from build123d import *

# Parameters (mm, degrees)
SKIZZE1_W                       = 63
SKIZZE1_H                       = 54
AUFSATZ_LINEAR_AUSTRAGEN1_DEPTH = 4
SCHNITT_LINEAR_AUSTRAGEN3_REACH = 6
SKIZZE4_W                       = 9.5
SKIZZE4_H                       = 4
SKIZZE2_W                       = 5
SKIZZE2_H                       = 17.25
SKIZZE2_H_2                     = 21.25
SCHNITT_LINEAR_AUSTRAGEN1_DEPTH = 4
SKIZZE5_R                       = 8
SCHNITT_LINEAR_AUSTRAGEN4_DEPTH = 4


with BuildPart() as part:
    # Skizze1 → Aufsatz-Linear austragen1 (new body)
    with BuildSketch(Plane.XY):
        with Locations((31.5, 27)):
            Rectangle(SKIZZE1_W, SKIZZE1_H)
    extrude(amount=AUFSATZ_LINEAR_AUSTRAGEN1_DEPTH)

    # Skizze4 → Schnitt-Linear austragen3 (cut, up to next)
    with BuildSketch(Plane.XY.offset(4), mode=Mode.PRIVATE) as schnitt_linear_austragen3_sk1:
        with Locations((19.669225385, 2)):
            Rectangle(SKIZZE4_W, SKIZZE4_H)
    schnitt_linear_austragen3_tool1 = extrude(schnitt_linear_austragen3_sk1.sketch, amount=-SCHNITT_LINEAR_AUSTRAGEN3_REACH, mode=Mode.PRIVATE) & part.part
    add(schnitt_linear_austragen3_tool1.solids().sort_by_distance((19.669225, 2, 4))[0], mode=Mode.SUBTRACT)
    # Skizze4 → Schnitt-Linear austragen3 (cut, up to next)
    with BuildSketch(Plane.XY.offset(4), mode=Mode.PRIVATE) as schnitt_linear_austragen3_sk2:
        with Locations((42.669225385, 2)):
            Rectangle(SKIZZE4_W, SKIZZE4_H)
    schnitt_linear_austragen3_tool2 = extrude(schnitt_linear_austragen3_sk2.sketch, amount=-SCHNITT_LINEAR_AUSTRAGEN3_REACH, mode=Mode.PRIVATE) & part.part
    add(schnitt_linear_austragen3_tool2.solids().sort_by_distance((42.669225, 2, 4))[0], mode=Mode.SUBTRACT)

    # Skizze2 → Schnitt-Linear austragen1 (cut)
    with BuildSketch(Plane.XY.offset(4)):
        with Locations((2.5, 45.375)):
            Rectangle(SKIZZE2_W, SKIZZE2_H)
        with Locations((2.5, 10.625)):
            Rectangle(SKIZZE2_W, SKIZZE2_H_2)
    schnitt_linear_austragen1 = extrude(amount=-SCHNITT_LINEAR_AUSTRAGEN1_DEPTH, mode=Mode.SUBTRACT)

    # Spiegeln1: Schnitt-Linear austragen1 across plane
    add(schnitt_linear_austragen1.mirror(Plane.ZY.offset(-31.5)), mode=Mode.SUBTRACT)

    # Skizze5 → Schnitt-Linear austragen4 (cut)
    with BuildSketch(Plane.XY.offset(4)):
        with Locations((18, 34)):
            Circle(SKIZZE5_R)
        with BuildLine():
            Line((31.5, 43.55), (28.2, 43.55))
            ThreePointArc((28.2, 43.55), (26.2, 41.55), (28.2, 39.55))
            Line((28.2, 39.55), (31.5, 39.55))
            Line((31.5, 39.55), (31.5, 43.55))
        make_face()
    schnitt_linear_austragen4 = extrude(amount=-SCHNITT_LINEAR_AUSTRAGEN4_DEPTH, mode=Mode.SUBTRACT)

    # Spiegeln2: Schnitt-Linear austragen4 across plane
    add(schnitt_linear_austragen4.mirror(Plane.ZY.offset(-31.5)), mode=Mode.SUBTRACT)


solid = part.part
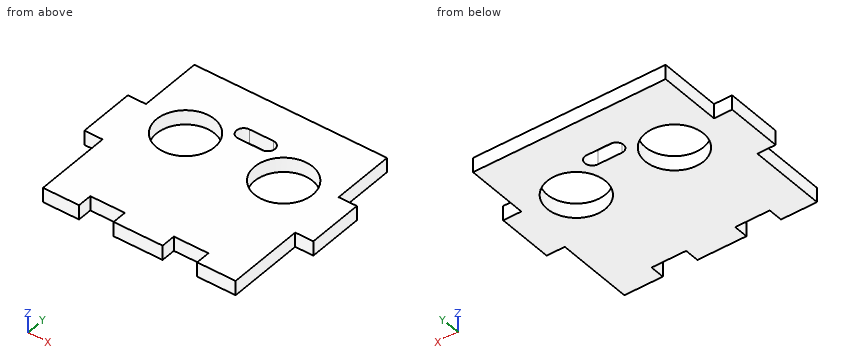
Part model, mm, in its own coordinate system. Give positions to 0.01 mm unless a question says otherwise; leave off trailing zeros. Loops run counter-clockwise (first coordinate to the right, second up) from the corner with the lowest first, then second, coordinate; pieces in that order, holes last. Notation, with made-up numbers: (-33, 77) -> (13, 77) arc R32 cw to (13, 111) -> close; hole circle Ø4 at (19, 0). An arc over 180 degrees is marked (long way). Write each question's results on one line, items separated by ' | '. Start each with the question number.
Q1. Band-saw the part on A-A on y = 34. List the corners of the cut face in (x, z).
Q2. Band-saw the part on D-D on x = 43.5. List the corners of the cut face in (y, z), plus the area to 3 significant figures.
Q3. Pin check, flat tips, straight feed: P1, Ø1.2, axis at y = 10, z = 2.5, coming from the -X side; P2, Ø2, axis at x = 17.5, z = 3, coming from the -Y side; P3, Ø1, axis at x = 51.5, y = 33, coming from the +Z side; P4, Ø2, axis at x = 3.5, z = 2.5, coming from the +Y side. Stop position of each tip, or through.
Q4. Wall check: L1, parallel to Y at x = 18, z = 2.3; L2, parallel to X at y = 31.5, z = 2.6; L3, parallel to X at y = 51.5, z = 0.2. Give the ranges that are in metal, low to high.
Q5. Band-saw the part on B-B on x = 18. List the corners of the cut face in (y, z), plus the area to 3 significant figures.
Q6. Band-saw the part on C-C on z = 1.75. List the corners of the cut face in (x, y).
Results are:
1) outline: (0, 0) -> (10, 0) -> (10, 4) -> (0, 4) -> close; (26, 0) -> (37, 0) -> (37, 4) -> (26, 4) -> close; (53, 0) -> (63, 0) -> (63, 4) -> (53, 4) -> close
2) outline: (4, 0) -> (26.14, 0) -> (26.14, 4) -> (4, 4) -> close; (41.86, 0) -> (54, 0) -> (54, 4) -> (41.86, 4) -> close | area: 137 mm²
3) P1: stops at x = 5 | P2: stops at y = 4 | P3: passes through | P4: stops at y = 36.75
4) L1: y = 4 to 26, 42 to 54 | L2: x = 0 to 10.4, 25.6 to 37.4, 52.6 to 63 | L3: x = 5 to 58
5) outline: (4, 0) -> (26, 0) -> (26, 4) -> (4, 4) -> close; (42, 0) -> (54, 0) -> (54, 4) -> (42, 4) -> close | area: 136 mm²
6) outline: (0, 21.25) -> (5, 21.25) -> (5, 0) -> (14.92, 0) -> (14.92, 4) -> (24.42, 4) -> (24.42, 0) -> (37.92, 0) -> (37.92, 4) -> (47.42, 4) -> (47.42, 0) -> (58, 0) -> (58, 21.25) -> (63, 21.25) -> (63, 36.75) -> (58, 36.75) -> (58, 54) -> (5, 54) -> (5, 36.75) -> (0, 36.75) -> close; hole circle Ø16 at (18, 34); hole (28.2, 39.55) -> (34.8, 39.55) arc R2 ccw to (34.8, 43.55) -> (28.2, 43.55) arc R2 ccw to start; hole circle Ø16 at (45, 34)
